For this review, take the finished solid that the model builds, in its own axes (mm). A direction names the side the tool comes from. Coordinates: 2 decimals unless noted, no trailing zeros. Write each loop counter-clockwise with the first axis right and the second up, starting at its lowest first coordinate (ties: lowest second). Pieces come first, ordered by that corner, then holes.
```python
from build123d import *

# Parameters (mm, degrees)
SKETCH1_W           = 20
SKETCH1_H           = 20
BOSS_EXTRUDE1_DEPTH = 3
FILLET1_R           = 1
SKETCH1_3_R         = 4
BOSS_EXTRUDE2_DEPTH = 5.75
SKETCH2_R           = 2.5
CUT_EXTRUDE1_DEPTH  = 5.75


with BuildPart() as part:
    # Sketch1 → Boss-Extrude1 (new body)
    with BuildSketch(Plane(origin=(0, 0, 0), x_dir=(1, 0, 0), z_dir=(0, 1, 0))):
        Rectangle(SKETCH1_W, SKETCH1_H)
    extrude(amount=BOSS_EXTRUDE1_DEPTH)

    # Fillet1
    fillet1_edges = [part.edges().sort_by_distance(p)[0] for p in [
        (-10, 1.5, -10),
        (-10, 1.5, 10),
        (10, 1.5, 10),
        (10, 1.5, -10),
    ]]
    fillet(fillet1_edges, radius=FILLET1_R)

    # Sketch1<3> → Boss-Extrude2 (add)
    with BuildSketch(Plane(origin=(0, 0, 0), x_dir=(1, 0, 0), z_dir=(0, 1, 0))):
        with Locations(Location((0, 0, 0), (0, 0, 90))):
            Circle(SKETCH1_3_R)
    extrude(amount=BOSS_EXTRUDE2_DEPTH)

    # Sketch2 → Cut-Extrude1 (cut)
    with BuildSketch(Plane(origin=(0, 5.75, 0), x_dir=(1, 0, 0), z_dir=(0, 1, 0))):
        with Locations(Location((0, 0, 0), (0, 0, 270))):
            Circle(SKETCH2_R)
    extrude(amount=-CUT_EXTRUDE1_DEPTH, mode=Mode.SUBTRACT)


solid = part.part
```
Q1. Add section D-D (z = 7). State the section outline as (x, y) points, then the cut area to 3 significant figures.
Ans:
outline: (-10, 0) - (10, 0) - (10, 3) - (-10, 3) - close
area: 60.0 mm2
Q2. Add section A-A (x = 0). State the section outline as (y, z) points.
Ans:
outline: (0, -10) - (3, -10) - (3, -4) - (5.75, -4) - (5.75, -2.5) - (0, -2.5) - close; (0, 2.5) - (5.75, 2.5) - (5.75, 4) - (3, 4) - (3, 10) - (0, 10) - close
Q3. Add section B-B (y = 2.05). State the section outline as (x, z) points, then the cut area to 3 significant figures.
Ans:
outline: (-10, -9) arc R1 ccw to (-9, -10) - (9, -10) arc R1 ccw to (10, -9) - (10, 9) arc R1 ccw to (9, 10) - (-9, 10) arc R1 ccw to (-10, 9) - close; hole circle Ø5 at (0, 0)
area: 380 mm2
Q4. Add section C-C (z = 0). State the section outline as (x, y) points.
Ans:
outline: (-10, 0) - (-2.5, 0) - (-2.5, 5.75) - (-4, 5.75) - (-4, 3) - (-10, 3) - close; (2.5, 0) - (10, 0) - (10, 3) - (4, 3) - (4, 5.75) - (2.5, 5.75) - close
Q5. Clearance check with flat-ended pins moving along their axes: pin 1 Ø6 at (x, z) = (-6.5, -6.5) entering from +Y; pin 2 Ø1.5 at (y, z) = (4, -2.5) entering from -X. State where each tip first meets the part, or that it passes through.
Ans:
pin 1: stops at y = 3
pin 2: stops at x = -3.6
Q6. Draft analysis for pull direction X (two halves, no side actions). For faces 1 (the cylindrical face through (-2.44, 2.92, -0.54)), 2 (the cylindrical face through (9.699, 1.521, 9.715)), 3 (the cylindrical face through (-9.715, 1.521, -9.699)), 4 (the flat face through (4.3, 3, -0.1)), state which applies: +X half, -X half, draft (parallel to the pull), parting line (faces both ways), or undercut.
Ans:
face 1: undercut
face 2: +X half
face 3: -X half
face 4: draft
Q7. Tool access review of faces 5 (the flat face through (-10, 1, 0)), 6 (the cylindrical face through (3.905, 4.356, 0.867)): name each direction out of +Z, -Z, +X, -X, +Y, -Y from which nothing blocks a thin tool from reaching the whole face with its end or side.
Ans:
face 5: +Z, -Z, -X, +Y, -Y
face 6: +Y
Q8. For probe 1 along X at (y, z) = (3.7, 0); probe 2 along X at (y, z) = (2.5, 0); probe 3 along Y at (x, z) = (-2.25, -4.5), list the stretches that pass through material, from the lowest coordinate up.
Ans:
probe 1: x = -4 to -2.5, 2.5 to 4
probe 2: x = -10 to -2.5, 2.5 to 10
probe 3: y = 0 to 3
